```python
from build123d import *

# Parameters (mm, degrees)
SKETCH1_W               = 80
SKETCH1_H               = 60
BOSS_EXTRUDE1_DEPTH     = 2.5
CUT_EXTRUDE4_DEPTH      = 51.062460986
CUT_EXTRUDE4_DEPTH_BACK = 51.062460986
SKETCH2_R               = 1.6
SKETCH3_W               = 2.5
SKETCH3_H               = 20.5
BOSS_EXTRUDE2_DEPTH     = 66.5
SKETCH4_W               = 80
SKETCH4_H               = 5.5
BOSS_EXTRUDE3_DEPTH     = 2.5
SKETCH5_W               = 2.5
SKETCH5_H               = 5.5
BOSS_EXTRUDE4_DEPTH     = 66.5
SKETCH6_W               = 2.5
SKETCH6_H               = 5.5
CUT_EXTRUDE5_DEPTH      = 66.5
SKETCH9_W               = 2.5
SKETCH9_H               = 2.5
BOSS_EXTRUDE5_DEPTH     = 66.5
SKETCH11_R              = 4.75
CUT_EXTRUDE6_DEPTH      = 2.5
SKETCH15_W              = 2.5
SKETCH15_H              = 23
BOSS_EXTRUDE6_DEPTH     = 8
SKETCH17_W              = 2.5
SKETCH17_H              = 74.5
BOSS_EXTRUDE7_DEPTH     = 2
SKETCH18_R              = 1.6
CUT_EXTRUDE7_DEPTH      = 2.5
SKETCH21_W              = 80
SKETCH21_H              = 2.5
BOSS_EXTRUDE8_DEPTH     = 2
SKETCH22_W              = 4.25
SKETCH22_H              = 74.5
CUT_EXTRUDE8_DEPTH      = 2.5
FILLET1_R               = 5
SKETCH23_W              = 15.225
SKETCH23_H              = 67.5
BOSS_EXTRUDE10_DEPTH    = 2.5
SKETCH24_W              = 95.225
SKETCH24_H              = 10
CUT_EXTRUDE9_DEPTH      = 101.031498164
SKETCH26_W              = 2.5
SKETCH26_H              = 20.75
BOSS_EXTRUDE11_DEPTH    = 74.5
SKETCH27_R              = 1.6
CUT_EXTRUDE10_DEPTH     = 2.5
SKETCH28_W              = 2.5
SKETCH28_H              = 20.75
CUT_EXTRUDE11_DEPTH     = 74.5
SKETCH29_W              = 20.75
SKETCH29_H              = 19.625
CUT_EXTRUDE12_DEPTH     = 2.5
FILLET2_R               = 6
SKETCH31_W              = 13.325
SKETCH31_H              = 57.5
CUT_EXTRUDE13_DEPTH     = 2.5
SKETCH33_W              = 3
SKETCH33_H              = 57.5
CUT_EXTRUDE14_DEPTH     = 2.5


with BuildPart() as part:
    # Sketch1 → Boss-Extrude1 (new body)
    with BuildSketch(Plane(origin=(0, 0, 0), x_dir=(1, 0, 0), z_dir=(0, 1, 0))):
        Rectangle(SKETCH1_W, SKETCH1_H)
    extrude(amount=BOSS_EXTRUDE1_DEPTH)

    # Sketch2 → Cut-Extrude4 (cut, two sides: drawn at the far end of the back side and taken through both)
    with BuildSketch(Plane(origin=(0, 0, 0), x_dir=(1, 0, 0), z_dir=(0, 1, 0)).offset(-CUT_EXTRUDE4_DEPTH_BACK)):
        with BuildLine():
            Line((-6.25, -24), (-2.5, -24))
            ThreePointArc((-2.5, -24), (0, -21.5), (2.5, -24))
            Line((2.5, -24), (16.25, -24))
            Line((16.25, -24), (16.25, -18))
            Line((16.25, -18), (-6.25, -18))
            Line((-6.25, -18), (-6.25, -24))
        make_face()
        with BuildLine():
            Line((0, -26.5), (0, -30))
            Line((0, -30), (16.25, -30))
            Line((16.25, -30), (16.25, -24))
            Line((16.25, -24), (2.5, -24))
            ThreePointArc((2.5, -24), (1.767766953, -25.767766953), (0, -26.5))
        make_face()
        with BuildLine():
            ThreePointArc((-2.5, -24), (-1.767766953, -25.767766953), (0, -26.5))
            Line((0, -26.5), (0, -24))
            Line((0, -24), (-2.5, -24))
        make_face()
        with BuildLine():
            Line((0, -24), (0, -26.5))
            ThreePointArc((0, -26.5), (1.767766953, -25.767766953), (2.5, -24))
            Line((2.5, -24), (0, -24))
        make_face()
        with BuildLine():
            Line((-2.5, -24), (0, -24))
            Line((0, -24), (2.5, -24))
            ThreePointArc((2.5, -24), (0, -21.5), (-2.5, -24))
        make_face()
        with BuildLine():
            ThreePointArc((-2.5, -24), (-1.767766953, -25.767766953), (0, -26.5))
            Line((0, -26.5), (0, -24))
            Line((0, -24), (-2.5, -24))
        make_face()
        with BuildLine():
            Line((0, -24), (0, -26.5))
            ThreePointArc((0, -26.5), (1.767766953, -25.767766953), (2.5, -24))
            Line((2.5, -24), (0, -24))
        make_face()
        with BuildLine():
            Line((-6.25, -30), (0, -30))
            Line((0, -30), (0, -26.5))
            ThreePointArc((0, -26.5), (-1.767766953, -25.767766953), (-2.5, -24))
            Line((-2.5, -24), (-6.25, -24))
            Line((-6.25, -24), (-6.25, -30))
        make_face()
        with Locations(Location((-8.625, -24, 0), (0, 0, 270))):
            Circle(SKETCH2_R)
        with Locations(Location((18.625, -24, 0), (0, 0, 270))):
            Circle(SKETCH2_R)
    extrude(amount=CUT_EXTRUDE4_DEPTH + CUT_EXTRUDE4_DEPTH_BACK, mode=Mode.SUBTRACT)

    # Sketch3 → Boss-Extrude2 (add)
    with BuildSketch(Plane(origin=(0, 2.5, 0), x_dir=(1, 0, 0), z_dir=(0, 1, 0))):
        with Locations((-38.75, -19.75)):
            Rectangle(SKETCH3_W, SKETCH3_H)
    extrude(amount=BOSS_EXTRUDE2_DEPTH)

    # Sketch4 → Boss-Extrude3 (add)
    with BuildSketch(Plane(origin=(0, 2.5, 0), x_dir=(1, 0, 0), z_dir=(0, 1, 0))):
        with Locations((0, -32.75)):
            Rectangle(SKETCH4_W, SKETCH4_H)
    extrude(amount=-BOSS_EXTRUDE3_DEPTH)

    # Sketch5 → Boss-Extrude4 (add)
    with BuildSketch(Plane(origin=(0, 2.5, 0), x_dir=(1, 0, 0), z_dir=(0, 1, 0))):
        with Locations((-38.75, -32.75)):
            Rectangle(SKETCH5_W, SKETCH5_H)
    extrude(amount=BOSS_EXTRUDE4_DEPTH)

    # Sketch6 → Cut-Extrude5 (cut)
    with BuildSketch(Plane(origin=(0, 69, 0), x_dir=(1, 0, 0), z_dir=(0, 1, 0))):
        with Locations((-38.75, -12.25)):
            Rectangle(SKETCH6_W, SKETCH6_H)
    extrude(amount=-CUT_EXTRUDE5_DEPTH, mode=Mode.SUBTRACT)

    # Sketch9 → Boss-Extrude5 (add)
    with BuildSketch(Plane(origin=(0, 2.5, 0), x_dir=(1, 0, 0), z_dir=(0, 1, 0))):
        with Locations((-38.75, -13.75)):
            Rectangle(SKETCH9_W, SKETCH9_H)
    extrude(amount=BOSS_EXTRUDE5_DEPTH)

    # Sketch11 → Cut-Extrude6 (cut)
    with BuildSketch(Plane(origin=(-37.5, 0, 0), x_dir=(0, 0, -1), z_dir=(1, 0, 0))):
        with Locations((-24, 54)):
            Circle(SKETCH11_R)
    extrude(amount=-CUT_EXTRUDE6_DEPTH, mode=Mode.SUBTRACT)

    # Sketch15 → Boss-Extrude6 (add)
    with BuildSketch(Plane(origin=(0, 69, 0), x_dir=(1, 0, 0), z_dir=(0, 1, 0))):
        with Locations((-38.75, -24)):
            Rectangle(SKETCH15_W, SKETCH15_H)
    extrude(amount=BOSS_EXTRUDE6_DEPTH)

    # Sketch17 → Boss-Extrude7 (add)
    with BuildSketch(Plane.XY.offset(35.5)):
        with Locations((-38.75, 39.75)):
            Rectangle(SKETCH17_W, SKETCH17_H)
    extrude(amount=BOSS_EXTRUDE7_DEPTH)

    # Sketch18 → Cut-Extrude7 (cut)
    with BuildSketch(Plane.ZY.offset(40)):
        with Locations((32, 36.5)):
            Circle(SKETCH18_R)
        with Locations((32, 71.5)):
            Circle(SKETCH18_R)
    extrude(amount=-CUT_EXTRUDE7_DEPTH, mode=Mode.SUBTRACT)

    # Sketch21 → Boss-Extrude8 (add)
    with BuildSketch(Plane.XY.offset(35.5)):
        with Locations((0, 1.25)):
            Rectangle(SKETCH21_W, SKETCH21_H)
    extrude(amount=BOSS_EXTRUDE8_DEPTH)

    # Sketch22 → Cut-Extrude8 (cut)
    with BuildSketch(Plane(origin=(-37.5, 0, 0), x_dir=(0, 0, -1), z_dir=(1, 0, 0))):
        with Locations((-14.625, 39.75)):
            Rectangle(SKETCH22_W, SKETCH22_H)
    extrude(amount=-CUT_EXTRUDE8_DEPTH, mode=Mode.SUBTRACT)

    # Fillet1
    fillet1_edges = [part.edges().sort_by_distance(p)[0] for p in [
        (-38.75, 77, 37.5),
        (-38.75, 77, 16.75),
    ]]
    fillet(fillet1_edges, radius=FILLET1_R)

    # Sketch23 → Boss-Extrude10 (add)
    with BuildSketch(Plane(origin=(0, 2.5, 0), x_dir=(1, 0, 0), z_dir=(0, 1, 0))):
        with Locations((47.6125, -3.75)):
            Rectangle(SKETCH23_W, SKETCH23_H)
    extrude(amount=-BOSS_EXTRUDE10_DEPTH)

    # Sketch24 → Cut-Extrude9 (cut, through all)
    with BuildSketch(Plane(origin=(0, 2.5, 0), x_dir=(1, 0, 0), z_dir=(0, 1, 0))):
        with Locations((7.6125, 25)):
            Rectangle(SKETCH24_W, SKETCH24_H)
    extrude(amount=-CUT_EXTRUDE9_DEPTH, mode=Mode.SUBTRACT)

    # Sketch26 → Boss-Extrude11 (add)
    with BuildSketch(Plane(origin=(0, 2.5, 0), x_dir=(1, 0, 0), z_dir=(0, 1, 0))):
        with Locations((-25.425, -27.125)):
            Rectangle(SKETCH26_W, SKETCH26_H)
    extrude(amount=BOSS_EXTRUDE11_DEPTH)

    # Sketch27 → Cut-Extrude10 (cut)
    with BuildSketch(Plane(origin=(-24.175, 0, 0), x_dir=(0, 0, -1), z_dir=(1, 0, 0))):
        with BuildLine():
            ThreePointArc((-28.75, 36.275), (-27.358757211, 32.916242789), (-24, 31.525))
            Line((-24, 31.525), (-24, 36.275))
            Line((-24, 36.275), (-28.75, 36.275))
        make_face()
        with BuildLine():
            Line((-24, 36.275), (-24, 31.525))
            ThreePointArc((-24, 31.525), (-20.641242789, 32.916242789), (-19.25, 36.275))
            ThreePointArc((-19.25, 36.275), (-24, 41.025), (-28.75, 36.275))
            Line((-28.75, 36.275), (-24, 36.275))
        make_face()
        with BuildLine():
            ThreePointArc((-28.75, 36.275), (-27.358757211, 32.916242789), (-24, 31.525))
            Line((-24, 31.525), (-24, 36.275))
            Line((-24, 36.275), (-28.75, 36.275))
        make_face()
        with BuildLine():
            Line((-24, 36.275), (-24, 31.525))
            ThreePointArc((-24, 31.525), (-20.641242789, 32.916242789), (-19.25, 36.275))
            ThreePointArc((-19.25, 36.275), (-24, 41.025), (-28.75, 36.275))
            Line((-28.75, 36.275), (-24, 36.275))
        make_face()
        with Locations((-32, 18.775)):
            Circle(SKETCH27_R)
        with Locations((-32, 53.775)):
            Circle(SKETCH27_R)
    extrude(amount=-CUT_EXTRUDE10_DEPTH, mode=Mode.SUBTRACT)

    # Sketch28 → Cut-Extrude11 (cut)
    with BuildSketch(Plane(origin=(0, 77, 0), x_dir=(1, 0, 0), z_dir=(0, 1, 0))):
        with Locations((-38.75, -27.125)):
            Rectangle(SKETCH28_W, SKETCH28_H)
    extrude(amount=-CUT_EXTRUDE11_DEPTH, mode=Mode.SUBTRACT)

    # Sketch29 → Cut-Extrude12 (cut)
    with BuildSketch(Plane(origin=(-24.175, 0, 0), x_dir=(0, 0, -1), z_dir=(1, 0, 0))):
        with Locations((-27.125, 67.1875)):
            Rectangle(SKETCH29_W, SKETCH29_H)
    extrude(amount=-CUT_EXTRUDE12_DEPTH, mode=Mode.SUBTRACT)

    # Fillet2
    fillet2_edges = [part.edges().sort_by_distance(p)[0] for p in [
        (-25.425, 57.375, 37.5),
        (-25.425, 57.375, 16.75),
    ]]
    fillet(fillet2_edges, radius=FILLET2_R)

    # Sketch31 → Cut-Extrude13 (cut)
    with BuildSketch(Plane(origin=(0, 2.5, 0), x_dir=(1, 0, 0), z_dir=(0, 1, 0))):
        with Locations((-33.3375, -8.75)):
            Rectangle(SKETCH31_W, SKETCH31_H)
    extrude(amount=-CUT_EXTRUDE13_DEPTH, mode=Mode.SUBTRACT)

    # Sketch33 → Cut-Extrude14 (cut)
    with BuildSketch(Plane(origin=(0, 2.5, 0), x_dir=(1, 0, 0), z_dir=(0, 1, 0))):
        with Locations((53.725, -8.75)):
            Rectangle(SKETCH33_W, SKETCH33_H)
    extrude(amount=-CUT_EXTRUDE14_DEPTH, mode=Mode.SUBTRACT)


solid = part.part
```
For this review, take the finished solid that the model builds, in its own axes (mm). A direction names the side the tool comes from. Round coordinates to 2 decimals unless told otherwise and drop trailing zeros. Order: outer loops, then holes, each group sorted by start corner. A loop starts at its lowest first (then second) coordinate and runs counter-clockwise, first axis right, second up.
Q1. We need section A-A, the plane x = 11. Give the boundary of the cut face in (y, z).
Findings below:
outline: (0, -20) - (2.5, -20) - (2.5, 18) - (0, 18) - close; (0, 30) - (2.5, 30) - (2.5, 37.5) - (0, 37.5) - close
Q2. We need section C-C, the plane y = 15. Give the boundary of the cut face in (x, z) (3 decimals), plus the area to 3 significant figures.
Findings below:
outline: (-26.675, 16.75) - (-24.175, 16.75) - (-24.175, 37.5) - (-26.675, 37.5) - close
area: 51.9 mm2
Q3. We need section D-D, the plane x = 43. Give the boundary of the cut face in (y, z).
Findings below:
outline: (0, -20) - (2.5, -20) - (2.5, 37.5) - (0, 37.5) - close
Q4. We need section B-B, the plane z = 27. Give the boundary of the cut face in (x, y) (3 decimals).
Findings below:
outline: (-26.675, 0) - (-6.25, 0) - (-6.25, 2.5) - (-24.175, 2.5) - (-24.175, 32.592) - (-26.675, 32.592) - close; (-26.675, 39.958) - (-24.175, 39.958) - (-24.175, 57.375) - (-26.675, 57.375) - close; (16.25, 0) - (52.225, 0) - (52.225, 2.5) - (16.25, 2.5) - close
Q5. Wall thickness on line 1 (X direction, y = 1.95, z = 24) (3 decimals); line 2 (Y direction, x = -25.15, z = 32) (3 decimals); line 3 (X direction, y = 30, z = 24) (3 decimals): over which ranges is each line inside the solid? List them lowest first.
Findings below:
line 1: x = -26.675 to -10.225, -7.025 to -6.25, 16.25 to 17.025, 20.225 to 52.225
line 2: y = 0 to 17.175, 20.375 to 52.175, 55.375 to 57.354
line 3: x = -26.675 to -24.175
Q6. Insertion check: P1, Ø3.5, axis at x = -8.625, z = 24, coming from the +Y side; P2, Ø0.8, axis at x = -26, y = 18.5, coming from the -Z side; P3, Ø4, axis at y = 18.775, z = 32, coming from the +X side (3 decimals); P4, Ø5, axis at x = -1.5, z = -5.5, coming from the -Y side. Each pin has a flat end and moves straight along its axis. Give the tip position at first contact, or say it passes through.
Findings below:
P1: stops at y = 2.5
P2: stops at z = 16.75
P3: stops at x = -24.175
P4: stops at y = 0
Q7. Machinability: for faces 4 (the flat face through (-6.25, 1, 24)), 5 (the flat face through (52.225, 1, 9)), 6 (the flat face through (-24.175, 30, 27)), which of the approach directions +Z, -Z, +X, -X, +Y, -Y give a long, thin tool a straight path to every point of the face, cutting with its end or side? Answer none if there is none.
Findings below:
face 4: +Y, -Y
face 5: +Z, -Z, +X, +Y, -Y
face 6: +Z, -Z, +X, +Y
Q8. Mouldability with a two-part tool opening along X and no side actions: class faces 1 (the cylindrical face through (20.21, 1.23, 23.79)), 2 (the flat face through (-25, 27, 16.75)), 3 (the flat face through (-26.675, 26, 26)) as pulls with the +X half, pulls with the -X half, needs draft (parallel to the pull), parting line crosses it, or undercut.
Findings below:
face 1: undercut
face 2: needs draft
face 3: pulls with the -X half
